Could you check a few things on this model? Use its own coordinates, in mm. Face numbers are marked on the shaded views. A direction names the side the tool comes from. Coordinates: 2 decimals unless noted, no trailing zeros. Write each loop counter-clockwise with the first axis right and the second up, starting at its lowest first coordinate (ties: lowest second). Pieces come first, ordered by that corner, then holes. Notation, with made-up numbers: M 21,26 L 41,26 A27 ccw 41,54 Z; hole C 21.25,-9.75 d8. An arc over 180 degrees is marked long. Write item = value, one per line.
```python
from build123d import *

# Parameters (mm, degrees)
F1_DEPTH  = 48
F2_SIZE2  = 35
F2_SIZE   = 22
F3_R      = 8
F4_DEPTH  = 2
F5_R      = 2.1
F6_DEPTH  = 5
F7_W      = 40
F7_H      = 15
F8_DEPTH  = 15
F9_R      = 2.8537362448
F10_DEPTH = 2


with BuildPart() as f1:
    # F0 (on Top) → F1 (new body)
    with BuildSketch(Plane.XY):
        Polygon((-8.3140695912, -83.1016019511), (79.5110319718, -25.5537823968), (76.1251331804, 34.3506055007), (-17.6252912675, 81.6354647671), (-67.8110635892, 48.7509964503), (-61.8911448644, -55.9860702678), align=None)
    extrude(amount=F1_DEPTH)

    # F2
    f2_edges = [f1.edges().sort_by_distance(p)[0] for p in [
        (-35.102607, -69.543836, 48),
        (35.598481, -54.327692, 48),
        (77.818083, 4.398412, 48),
        (29.249921, 57.993035, 48),
        (-42.718177, 65.193231, 48),
        (-64.851104, -3.617537, 48),
    ]]
    chamfer(f2_edges, length=F2_SIZE, length2=F2_SIZE2)

    # F3 (on face) → F4 (cut)
    with BuildSketch(Plane.XY.offset(48)):
        with Locations((0, -1.6585105106)):
            Circle(F3_R)
    extrude(amount=-F4_DEPTH, mode=Mode.SUBTRACT)

    # F5 (on face) → F6 (cut)
    with BuildSketch(Plane(origin=(0, 0, 0), x_dir=(1, 0, 0), z_dir=(0, 0, -1))):
        with Locations((17.2813809108, 39.0870698365)):
            Circle(F5_R)
        with Locations((12.766849189, -40.7854473602)):
            Circle(F5_R)
    extrude(amount=-F6_DEPTH, mode=Mode.SUBTRACT)

    # F7 (on face) → F8 (cut)
    with BuildSketch(Plane(origin=(-64.8484021467, -3.66534296, 0), x_dir=(0.0564316465, -0.998406465, 0), z_dir=(-0.998406465, -0.0564316465, 0))):
        with Locations((0.5, 7.5)):
            Rectangle(F7_W, F7_H)
    extrude(amount=-F8_DEPTH, mode=Mode.SUBTRACT)

    # F9 (on face) → F10 (cut)
    with BuildSketch(Plane.XY.offset(48)):
        with Locations((26.1640120298, 0)):
            Circle(F9_R)
    extrude(amount=-F10_DEPTH, mode=Mode.SUBTRACT)


solid = f1.part
```
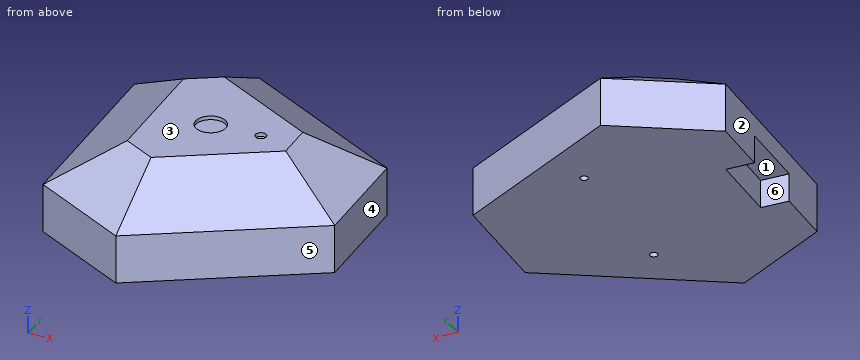
Item 1: I'm going to push flat-ended pins straight in: P1, Ø8, axis at x = -1, y = -5, coming from the +Z side; P2, Ø12, axis at x = -49.5, z = 18, coming from the -Y side; P3, Ø12, axis at x = -38, z = 19, coming from the +Y side. Where does each tip first touch, or does it pass through?
Numbers:
P1 = 46
P2 = -65.29
P3 = 72.22
Item 2: For the marked faces 5 and 6, which set-ups out of +Z, -Z, +X, -X, +Y, -Y let a thin tool reach every point of the face, with its end or its side?
Numbers:
face_5 = +Z, -Z, +X, -Y
face_6 = -Z, -X
Item 3: Imagine slicing it at B-B (y = -11.5). Write out the boundary of the cut face in (x, z).
Numbers:
outline = M -64.41,15 L -49.38,15 L -49.38,0 L 78.72,0 L 78.72,26 L 51.65,42.99 L 37.1,48 L -29.35,48 L -64.41,26 Z
Item 4: Imagine slicing it at C-C (x = -19.5). Write out the boundary of the cut face in (y, z).
Numbers:
outline = M -77.44,0 L 80.41,0 L 80.41,26 L 38.56,48 L -38.21,48 L -77.44,26 Z
Item 5: Imagine slicing it at D-D (z = 21). Write out the boundary of the cut face in (x, y).
Numbers:
outline = M -67.81,48.75 L -61.89,-55.99 L -8.31,-83.1 L 79.51,-25.55 L 76.13,34.35 L -17.63,81.64 Z
Item 6: Imagine slicing it at A-A (z = 11.5). Write out the boundary of the cut face in (x, y), and give its area (3 significant figures).
Numbers:
outline = M -67.81,48.75 L -65.95,15.8 L -50.97,16.65 L -48.72,-23.29 L -63.69,-24.13 L -61.89,-55.99 L -8.31,-83.1 L 79.51,-25.55 L 76.13,34.35 L -17.63,81.64 Z
area = 16,600 mm²
Item 7: If I drill on line 1 along Z through (x, y) = (-49, -43.5); line 2 along Y through (x, z) = (-3, 40); line 3 along Y through (x, z) = (-26, 10.5), over which ranges is the centre line in solid material (lowest first)?
Numbers:
line_1 = 0 to 34.53
line_2 = -52.99 to 49.31
line_3 = -74.15 to 76.15
Item 8: If we mould it in two halves opening along Y, with no side actions, what happens to the marked faces 1, 2, 3 and 4? For each: pulls with the +Y half, pulls with the -Y half, needs draft (parallel to the pull), parting line crosses it, or undercut.
Numbers:
face_1 = undercut
face_2 = pulls with the -Y half
face_3 = needs draft
face_4 = pulls with the +Y half
